```python
from build123d import *

# Parameters (mm, degrees)
IZIM1_W                     = 60
IZIM1_H                     = 43.037715622
IZIM1_W_2                   = 54
IZIM1_H_2                   = 37.037715622
Y_KSEKLIK_EKSTR_ZYON1_DEPTH = 110
IZIM2_W                     = 60
IZIM2_H                     = 20
KES_EKSTR_ZYON1_DEPTH       = 10
IZIM3_W                     = 60
IZIM3_H                     = 43.037715622
Y_KSEKLIK_EKSTR_ZYON2_DEPTH = 10
IZIM4_W                     = 60
IZIM4_H                     = 55
KES_EKSTR_ZYON2_DEPTH       = 70
IZIM5_W                     = 60
IZIM5_H                     = 43.037715622
Y_KSEKLIK_EKSTR_ZYON3_DEPTH = 5


with BuildPart() as part:
    # Çizim1 → Yükseklik-Ekstrüzyon1 (new body)
    with BuildSketch(Plane.XY):
        with Locations((30, 21.518857811)):
            Rectangle(IZIM1_W, IZIM1_H)
        with Locations((30, 21.518857811)):
            Rectangle(IZIM1_W_2, IZIM1_H_2, mode=Mode.SUBTRACT)
    extrude(amount=Y_KSEKLIK_EKSTR_ZYON1_DEPTH)

    # Çizim2 → Kes-Ekstrüzyon1 (cut)
    with BuildSketch(Plane(origin=(0, 43.037715622, 0), x_dir=(1, 0, 0), z_dir=(0, 1, 0))):
        with Locations((30, -10)):
            Rectangle(IZIM2_W, IZIM2_H)
    extrude(amount=-KES_EKSTR_ZYON1_DEPTH, mode=Mode.SUBTRACT)

    # Çizim3 → Yükseklik-Ekstrüzyon2 (add)
    with BuildSketch(Plane.XY.offset(110)):
        with Locations((30, 21.518857811)):
            Rectangle(IZIM3_W, IZIM3_H)
    extrude(amount=-Y_KSEKLIK_EKSTR_ZYON2_DEPTH)

    # Çizim4 → Kes-Ekstrüzyon2 (cut)
    with BuildSketch(Plane(origin=(0, 43.037715622, 0), x_dir=(1, 0, 0), z_dir=(0, 1, 0))):
        with Locations((30, -82.5)):
            Rectangle(IZIM4_W, IZIM4_H)
    extrude(amount=-KES_EKSTR_ZYON2_DEPTH, mode=Mode.SUBTRACT)

    # Çizim5 → Yükseklik-Ekstrüzyon3 (add)
    with BuildSketch(Plane.XY.offset(55)):
        with Locations((30, 21.518857811)):
            Rectangle(IZIM5_W, IZIM5_H)
    extrude(amount=-Y_KSEKLIK_EKSTR_ZYON3_DEPTH)


solid = part.part
```
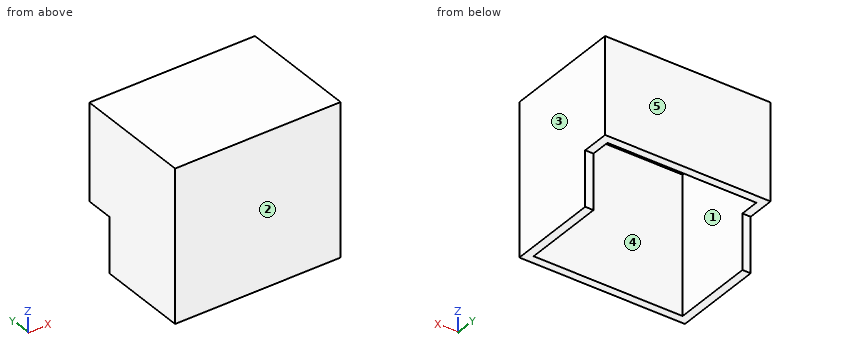
Can you work these out from the model? Positions are in its coordinate system, mm. Face numbers are marked on the shaded views. A direction names the side the tool comes from. Give positions to 0.01 mm unless a question says otherwise; leave off trailing zeros. Loops run counter-clockwise (first coordinate to the right, second up) from the corner with the lowest first, then second, coordinate; pieces in that order, holes last. Notation, with made-up numbers: M 12.5,-17.5 L 55.5,-17.5 A28 cw 55.5,0.5 Z; hole C 44.5,41.5 d5. An arc over 180 degrees is marked long. One line per question, with ' | ' between items. Start each with the question number.
Q1. If we mould it in two halves opening along Y, with no side actions, what happens to the marked faces 1, 2 and 3? For each: +Y half, -Y half, draft (parallel to the pull), parting line (faces both ways), or undercut.
Q2. If we section it at A-A (z = 41.5): Please give me the cut outline in (x, y), plus the area to 3 significant figures.
Q3. If we section it at B-B (x = 14.5): Please give me the cut outline in (y, z).
Q4. For the marked faces 4 and 5, which set-ups out of +Z, -Z, +X, -X, +Y, -Y let a thin tool reach every point of the face, with its end or its side?
Q5. For pin 1 Ø0.9 at (x, z) = (58.5, 12.5) entering from +Y; pin 2 Ø11 at (x, y) = (21, 36.5) entering from -Z; pin 3 Ø1.5 at (x, y) = (34, 16) entering from -Z, each with a flat end and sliding along its axis, tell me the tip position at first contact or that it passes through.
Q6. If we section it at C-C (z = 7): Please give me the cut outline in (x, y).
Q7. If I drill on line 1 (Y direction, x = 31.5, z = 37); line 2 (X direction, y = 30, z = 45); line 3 (Z direction, x = 30, y = 41), over which ranges is the centre line in solid material (lowest first)? Write a range as from..to.
Computed:
1) face 1: undercut | face 2: -Y half | face 3: draft
2) outline: M 0,0 L 60,0 L 60,43.04 L 0,43.04 Z; hole M 3,3 L 57,3 L 57,40.04 L 3,40.04 Z | area: 582 mm²
3) outline: M 0,0 L 3,0 L 3,50 L 40.04,50 L 40.04,20 L 43.04,20 L 43.04,55 L 0,55 Z
4) face 4: -Z | face 5: +Z, -Z, +X, -X, +Y
5) pin 1: stops at y = 33.04 | pin 2: stops at z = 20 | pin 3: stops at z = 50
6) outline: M 0,0 L 60,0 L 60,33.04 L 57,33.04 L 57,3 L 3,3 L 3,33.04 L 0,33.04 Z
7) line 1: y = 0..3, 40.04..43.04 | line 2: x = 0..3, 57..60 | line 3: z = 20..55
